Autodesk Inventor part; units mm, degrees
ref_plane "YZ Plane" through (0, 0, 0) normal (1, 0, 0) x (0, 1, 0)
ref_plane "XZ Plane" through (0, 0, 0) normal (0, 1, 0) x (-1, 0, 0)
ref_plane "XY Plane" through (0, 0, 0) normal (0, 0, 1) x (1, 0, 0)
sketch "Sketch1" plane through (0, 0, 0) normal (0, 1, 0) x (-1, 0, 0)
  line L0 (-9, 48) -> (-9, -48)
  line L1 (-7, -50) -> (7, -50)
  line L2 (9, -48) -> (9, 48)
  line L3 (7, 50) -> (-7, 50)
  line L4 (-9, 50) -> (9, -50) construction
  line L5 (-9, -50) -> (9, 50) construction
  arc A0 (9, 48) -> (7, 50) centre (7, 48) ccw
  arc A1 (-7, 50) -> (-9, 48) centre (-7, 48) ccw
  arc A2 (-9, -48) -> (-7, -50) centre (-7, -48) ccw
  arc A3 (7, -50) -> (9, -48) centre (7, -48) ccw
  line L6 (-7, 47) -> (-7, 47)
  line L7 (-6, 46) -> (6, 46)
  line L8 (7, 47) -> (7, 47)
  line L9 (6, 48) -> (-6, 48)
  arc A4 (7, 47) -> (6, 48) centre (6, 47) ccw
  arc A5 (6, 46) -> (7, 47) centre (6, 47) ccw
  arc A6 (-6, 48) -> (-7, 47) centre (-6, 47) ccw
  arc A7 (-7, 47) -> (-6, 46) centre (-6, 47) ccw
  line L10 (-7, 37.6) -> (-7, 37.6)
  line L11 (-6, 36.6) -> (6, 36.6)
  line L12 (7, 37.6) -> (7, 37.6)
  line L13 (6, 38.6) -> (-6, 38.6)
  arc A8 (7, 37.6) -> (6, 38.6) centre (6, 37.6) ccw
  arc A9 (6, 36.6) -> (7, 37.6) centre (6, 37.6) ccw
  arc A10 (-6, 38.6) -> (-7, 37.6) centre (-6, 37.6) ccw
  arc A11 (-7, 37.6) -> (-6, 36.6) centre (-6, 37.6) ccw
  line L14 (-7, 28.2) -> (-7, 28.2)
  line L15 (-6, 27.2) -> (6, 27.2)
  line L16 (7, 28.2) -> (7, 28.2)
  line L17 (6, 29.2) -> (-6, 29.2)
  arc A12 (7, 28.2) -> (6, 29.2) centre (6, 28.2) ccw
  arc A13 (6, 27.2) -> (7, 28.2) centre (6, 28.2) ccw
  arc A14 (-6, 29.2) -> (-7, 28.2) centre (-6, 28.2) ccw
  arc A15 (-7, 28.2) -> (-6, 27.2) centre (-6, 28.2) ccw
  line L18 (-7, 18.8) -> (-7, 18.8)
  line L19 (-6, 17.8) -> (6, 17.8)
  line L20 (7, 18.8) -> (7, 18.8)
  line L21 (6, 19.8) -> (-6, 19.8)
  arc A16 (7, 18.8) -> (6, 19.8) centre (6, 18.8) ccw
  arc A17 (6, 17.8) -> (7, 18.8) centre (6, 18.8) ccw
  arc A18 (-6, 19.8) -> (-7, 18.8) centre (-6, 18.8) ccw
  arc A19 (-7, 18.8) -> (-6, 17.8) centre (-6, 18.8) ccw
  line L22 (-7, 9.4) -> (-7, 9.4)
  line L23 (-6, 8.4) -> (6, 8.4)
  line L24 (7, 9.4) -> (7, 9.4)
  line L25 (6, 10.4) -> (-6, 10.4)
  arc A20 (7, 9.4) -> (6, 10.4) centre (6, 9.4) ccw
  arc A21 (6, 8.4) -> (7, 9.4) centre (6, 9.4) ccw
  arc A22 (-6, 10.4) -> (-7, 9.4) centre (-6, 9.4) ccw
  arc A23 (-7, 9.4) -> (-6, 8.4) centre (-6, 9.4) ccw
  line L26 (-7, 0) -> (-7, 0)
  line L27 (-6, -1) -> (6, -1)
  line L28 (7, 0) -> (7, 0)
  line L29 (6, 1) -> (-6, 1)
  arc A24 (7, 0) -> (6, 1) centre (6, 0) ccw
  arc A25 (6, -1) -> (7, 0) centre (6, 0) ccw
  arc A26 (-6, 1) -> (-7, 0) centre (-6, 0) ccw
  arc A27 (-7, 0) -> (-6, -1) centre (-6, 0) ccw
  line L30 (-7, -9.4) -> (-7, -9.4)
  line L31 (-6, -10.4) -> (6, -10.4)
  line L32 (7, -9.4) -> (7, -9.4)
  line L33 (6, -8.4) -> (-6, -8.4)
  arc A28 (7, -9.4) -> (6, -8.4) centre (6, -9.4) ccw
  arc A29 (6, -10.4) -> (7, -9.4) centre (6, -9.4) ccw
  arc A30 (-6, -8.4) -> (-7, -9.4) centre (-6, -9.4) ccw
  arc A31 (-7, -9.4) -> (-6, -10.4) centre (-6, -9.4) ccw
  line L34 (-7, -18.8) -> (-7, -18.8)
  line L35 (-6, -19.8) -> (6, -19.8)
  line L36 (7, -18.8) -> (7, -18.8)
  line L37 (6, -17.8) -> (-6, -17.8)
  arc A32 (7, -18.8) -> (6, -17.8) centre (6, -18.8) ccw
  arc A33 (6, -19.8) -> (7, -18.8) centre (6, -18.8) ccw
  arc A34 (-6, -17.8) -> (-7, -18.8) centre (-6, -18.8) ccw
  arc A35 (-7, -18.8) -> (-6, -19.8) centre (-6, -18.8) ccw
  line L38 (-7, -28.2) -> (-7, -28.2)
  line L39 (-6, -29.2) -> (6, -29.2)
  line L40 (7, -28.2) -> (7, -28.2)
  line L41 (6, -27.2) -> (-6, -27.2)
  arc A36 (7, -28.2) -> (6, -27.2) centre (6, -28.2) ccw
  arc A37 (6, -29.2) -> (7, -28.2) centre (6, -28.2) ccw
  arc A38 (-6, -27.2) -> (-7, -28.2) centre (-6, -28.2) ccw
  arc A39 (-7, -28.2) -> (-6, -29.2) centre (-6, -28.2) ccw
  line L42 (-7, -37.6) -> (-7, -37.6)
  line L43 (-6, -38.6) -> (6, -38.6)
  line L44 (7, -37.6) -> (7, -37.6)
  line L45 (6, -36.6) -> (-6, -36.6)
  arc A40 (7, -37.6) -> (6, -36.6) centre (6, -37.6) ccw
  arc A41 (6, -38.6) -> (7, -37.6) centre (6, -37.6) ccw
  arc A42 (-6, -36.6) -> (-7, -37.6) centre (-6, -37.6) ccw
  arc A43 (-7, -37.6) -> (-6, -38.6) centre (-6, -37.6) ccw
  line L46 (-7, -47) -> (-7, -47)
  line L47 (-6, -48) -> (6, -48)
  line L48 (7, -47) -> (7, -47)
  line L49 (6, -46) -> (-6, -46)
  arc A44 (7, -47) -> (6, -46) centre (6, -47) ccw
  arc A45 (6, -48) -> (7, -47) centre (6, -47) ccw
  arc A46 (-6, -46) -> (-7, -47) centre (-6, -47) ccw
  arc A47 (-7, -47) -> (-6, -48) centre (-6, -47) ccw
  point P0 (0, 0)
  point P1 (-7, 46)
  point P2 (7, 38.6)
  point P3 (-7, 38.6)
  point P4 (-7, 36.6)
  point P5 (7, 29.2)
  point P6 (-7, 29.2)
  point P7 (-7, 27.2)
  point P8 (7, 19.8)
  point P9 (-7, 19.8)
  point P10 (-7, 17.8)
  point P11 (7, 10.4)
  point P12 (-7, 10.4)
  point P13 (-7, 8.4)
  point P14 (7, 1)
  point P15 (-7, 1)
  point P16 (-7, -1)
  point P17 (7, -8.4)
  point P18 (-7, -8.4)
  point P19 (-7, -10.4)
  point P20 (7, -17.8)
  point P21 (-7, -17.8)
  point P22 (-7, -19.8)
  point P23 (7, -27.2)
  point P24 (-7, -27.2)
  point P25 (-7, -29.2)
  point P26 (7, -36.6)
  point P27 (-7, -36.6)
  point P28 (-7, -38.6)
  point P29 (7, -46)
  point P30 (-7, -46)
  point P31 (-7, -48)
  dimension "d0" = 100
  dimension "d1" = 18
  dimension "d2" = 2
  dimension "d3" = 2
  dimension "d4" = 1
  dimension "d5" = 1
  dimension "d8" = 9.4
extrude "Extrusion1" add sketch "Sketch1" along normal blind 2
properties part number "Kicker Plate"
Verification items for the finished model (mm, model axes). A direction names the side the tool comes from. Coordinates: 2 decimals unless noted, no trailing zeros. Loops run counter-clockwise (first coordinate to the right, second up) from the corner with the lowest first, then second, coordinate; pieces in that order, holes last. Notation, with made-up numbers: (-21, 89) - (-15, 89) arc R17 ccw to (-15, 100) - close; hole circle Ø11 at (46.25, 69.25). An arc over 180 degrees is marked (long way). Return JSON: item names as keys, results as strings.
1. Thickness scan on L1, parallel to X at y = 0.25, z = -9; L2, parallel to Z at x = 8.25, y = 1.15. Record the ranges inside material, lowest first.
Established:
{"L1": "x = -9 to -6.92, 6.92 to 9", "L2": "z = -49.56 to 49.56"}
2. Go/stop test with a flat-tipped pin: pin 1 (8 mm diameter, centred on x = -5, z = -27.5, fed in from +Y). Record where the tip stops, or that it passes through.
Established:
{"pin 1": "stops at y = 2"}
3. Tool access check on faces 1 (the cylindrical face through (7, 1, 18.8)), 2 (the cylindrical face through (-8.4, 0.99, 49.43)). Record the directions out of +Z, -Z, +X, -X, +Y, -Y that give a thin tool (end or side, any length) a straight path to the whole face; none if there is none.
Established:
{"face 1": "+Y, -Y", "face 2": "+Z, -X, +Y, -Y"}
4. Section check B-B, the plane x = -4. Count the separate pieces of the cut face and the enclosed holes in it, then the cut area to 3 significant figures.
Established:
{"separate pieces": "12", "enclosed holes": "0", "area": "156 mm2"}
5. Mould release check, pull along X, two halves, no side actions. Record for faces 3 (the cylindrical face through (-7, 1, 9.4)), 4 (the cylindrical face through (7, 1, 9.4)), 5 (the flat face through (0, 1, -50)), 6 (the cylindrical face through (-8.43, 0.99, -49.4)): +X half, -X half, draft (parallel to the pull), parting line (faces both ways), or undercut.
Established:
{"face 3": "undercut", "face 4": "undercut", "face 5": "draft", "face 6": "-X half"}
6. Section check A-A, the plane z = -9.4. Record the boundary of the cut face in (x, y).
Established:
{"outline": "(-9, 0) - (-7, 0) - (-7, 2) - (-9, 2) - close; (7, 0) - (9, 0) - (9, 2) - (7, 2) - close"}
